```python
from build123d import *

# Parameters (mm, degrees)
ESQUISSE1_W             = 190
ESQUISSE1_H             = 95
BOSS_EXTRU_1_DEPTH      = 6
ESQUISSE9_W             = 12.5
ESQUISSE9_H             = 7.5
ESQUISSE9_W_2           = 25
ESQUISSE9_W_3           = 7.5
ESQUISSE9_H_2           = 12.5
ESQUISSE9_H_3           = 25
ENL_V_MAT_EXTRU_1_DEPTH = 6


with BuildPart() as part:
    # Esquisse1 → Boss.-Extru.1 (new body)
    with BuildSketch(Plane(origin=(0, 0, 0), x_dir=(1, 0, 0), z_dir=(0, 1, 0))):
        with Locations((-95, -47.5)):
            Rectangle(ESQUISSE1_W, ESQUISSE1_H)
    extrude(amount=BOSS_EXTRU_1_DEPTH)

    # Esquisse9 → Enlèv. mat.-Extru.1 (cut)
    with BuildSketch(Plane(origin=(0, 6, 0), x_dir=(1, 0, 0), z_dir=(0, 1, 0))):
        with Locations((-183.75, -23.75)):
            Rectangle(ESQUISSE9_W, ESQUISSE9_H)
        with Locations((-142.5, -23.75)):
            Rectangle(ESQUISSE9_W_2, ESQUISSE9_H)
        with Locations((-183.75, -71.25)):
            Rectangle(ESQUISSE9_W, ESQUISSE9_H)
        with Locations((-142.5, -71.25)):
            Rectangle(ESQUISSE9_W_2, ESQUISSE9_H)
        with Locations((-95, -71.25)):
            Rectangle(ESQUISSE9_W_2, ESQUISSE9_H)
        with Locations((-95, -23.75)):
            Rectangle(ESQUISSE9_W_2, ESQUISSE9_H)
        with Locations((-47.5, -23.75)):
            Rectangle(ESQUISSE9_W_2, ESQUISSE9_H)
        with Locations((-6.25, -23.75)):
            Rectangle(ESQUISSE9_W, ESQUISSE9_H)
        with Locations((-47.5, -71.25)):
            Rectangle(ESQUISSE9_W_2, ESQUISSE9_H)
        with Locations((-6.25, -71.25)):
            Rectangle(ESQUISSE9_W, ESQUISSE9_H)
        with Locations((-166.25, -88.75)):
            Rectangle(ESQUISSE9_W_3, ESQUISSE9_H_2)
        with Locations((-166.25, -47.5)):
            Rectangle(ESQUISSE9_W_3, ESQUISSE9_H_3)
        with Locations((-166.25, -6.25)):
            Rectangle(ESQUISSE9_W_3, ESQUISSE9_H_2)
        with Locations((-118.75, -88.75)):
            Rectangle(ESQUISSE9_W_3, ESQUISSE9_H_2)
        with Locations((-71.25, -88.75)):
            Rectangle(ESQUISSE9_W_3, ESQUISSE9_H_2)
        with Locations((-23.75, -88.75)):
            Rectangle(ESQUISSE9_W_3, ESQUISSE9_H_2)
        with Locations((-118.75, -47.5)):
            Rectangle(ESQUISSE9_W_3, ESQUISSE9_H_3)
        with Locations((-71.25, -47.5)):
            Rectangle(ESQUISSE9_W_3, ESQUISSE9_H_3)
        with Locations((-23.75, -47.5)):
            Rectangle(ESQUISSE9_W_3, ESQUISSE9_H_3)
        with Locations((-118.75, -6.25)):
            Rectangle(ESQUISSE9_W_3, ESQUISSE9_H_2)
        with Locations((-71.25, -6.25)):
            Rectangle(ESQUISSE9_W_3, ESQUISSE9_H_2)
        with Locations((-23.75, -6.25)):
            Rectangle(ESQUISSE9_W_3, ESQUISSE9_H_2)
    extrude(amount=-ENL_V_MAT_EXTRU_1_DEPTH, mode=Mode.SUBTRACT)


solid = part.part
```
Geometry: final body of the model. Coordinates: model frame, mm. A direction names the side the tool comes from. Give positions to 0.01 mm unless a question says otherwise; leave off trailing zeros. Loops run counter-clockwise (first coordinate to the right, second up) from the corner with the lowest first, then second, coordinate; pieces in that order, holes last. Notation, with made-up numbers: (45.25, 35) - (83.25, 35) arc R20 ccw to (83.25, 52) - close; hole circle Ø8 at (63.25, 86). An arc over 180 degrees is marked (long way). Answer as CSV lines item,"result". Start each with the question number.
(1) Reachability of faces 1 (the face through (-143, 3, 27.5)), 2 (the face through (-27.5, 3, 6)), 3 (the face through (-177.5, 3, 71)) from +Z, -Z, +X, -X, +Y, -Y: full face, straight path, thin tool, end or side. Return the list, or none.
(2) Section query A-A (z = 10.5). Output: boundary loops of the cut face in (x, y), and give its area (3 significant figures).
(3) Mould query, pull axis Z, two halves, no side actions, for faces 4 (the face through (-180, 3, 0)), 5 (the face through (-190, 3, 85)), 6 (the face through (-60, 3, 71)). Classes: +Z half, -Z half, draft (parallel to the pull), parting line (faces both ways), or undercut.
(4) Section query B-B (x = -146). Output: boundary loops of the cut face in (y, z).
(5) Pin query (flat end, axial travel): P1, Ø4, axis at x = -30, z = 19, coming from the -Y side; P2, Ø3, axis at y = 4, z = 23.5, coming from the -X side; P3, Ø1.8, axis at x = -70.5, y = 3, coming from the +Z side. Return the tip coordinate at first contact, or that it passes through.
(6) Section query C-C (y = 2.75). Give the number of separate pieces and of enclosed holes in the cut face, and give its area (4 significant figures).
(7) Ray query, line 1 along Z through (x, y) = (-56, 3.3); line 2 along X through (y, z) = (1.85, 9.5); line 3 along X through (y, z) = (2.5, 74). Return the intervals inside material, ascending. Write a range as [from, to].
Worked answers:
1,face 1,"+Y, -Y"
1,face 2,"-Z, +Y, -Y"
1,face 3,"-X, +Y, -Y"
2,outline,"(-190, 0) - (-170, 0) - (-170, 6) - (-190, 6) - close; (-162.5, 0) - (-122.5, 0) - (-122.5, 6) - (-162.5, 6) - close; (-115, 0) - (-75, 0) - (-75, 6) - (-115, 6) - close; (-67.5, 0) - (-27.5, 0) - (-27.5, 6) - (-67.5, 6) - close; (-20, 0) - (0, 0) - (0, 6) - (-20, 6) - close"
2,area,"960 mm^2"
3,face 4,"-Z half"
3,face 5,"draft"
3,face 6,"undercut"
4,outline,"(0, 0) - (6, 0) - (6, 20) - (0, 20) - close; (0, 27.5) - (6, 27.5) - (6, 67.5) - (0, 67.5) - close; (0, 75) - (6, 75) - (6, 95) - (0, 95) - close"
5,P1,"stops at y = 0"
5,P2,"stops at x = -177.5"
5,P3,"stops at z = 82.5"
6,separate pieces,"1"
6,enclosed holes,"10"
6,area,"15,050 mm^2"
7,line 1,"z = [0, 20], [27.5, 67.5], [75, 95]"
7,line 2,"x = [-190, -170], [-162.5, -122.5], [-115, -75], [-67.5, -27.5], [-20, 0]"
7,line 3,"x = [-177.5, -155], [-130, -107.5], [-82.5, -60], [-35, -12.5]"
